```python
from build123d import *

# Parameters (mm, degrees)
CROQUIS1_R              = 2.5
SALIENTE_EXTRUIR1_DEPTH = 62
CORTAR_EXTRUIR1_DEPTH   = 17.5
CHAFL_N1_SIZE           = 0.2


with BuildPart() as part:
    # Croquis1 → Saliente-Extruir1 (new body)
    with BuildSketch(Plane(origin=(0, 0, 0), x_dir=(1, 0, 0), z_dir=(0, 1, 0))):
        Circle(CROQUIS1_R)
    extrude(amount=SALIENTE_EXTRUIR1_DEPTH)

    # Croquis2 → Cortar-Extruir1 (cut)
    with BuildSketch(Plane(origin=(0, 62, 0), x_dir=(1, 0, 0), z_dir=(0, 1, 0))):
        with BuildLine():
            Line((-1.920937271, 1.6), (1.920937271, 1.6))
            ThreePointArc((1.920937271, 1.6), (0, 2.5), (-1.920937271, 1.6))
        make_face()
    extrude(amount=-CORTAR_EXTRUIR1_DEPTH, mode=Mode.SUBTRACT)

    # Chaflán1
    chafl_n1_edges = [part.edges().sort_by_distance(p)[0] for p in [
        (-0.850781059, 62, 2.350781059),
        (-2.5, 0, 0),
    ]]
    chamfer(chafl_n1_edges, length=CHAFL_N1_SIZE)


solid = part.part
```
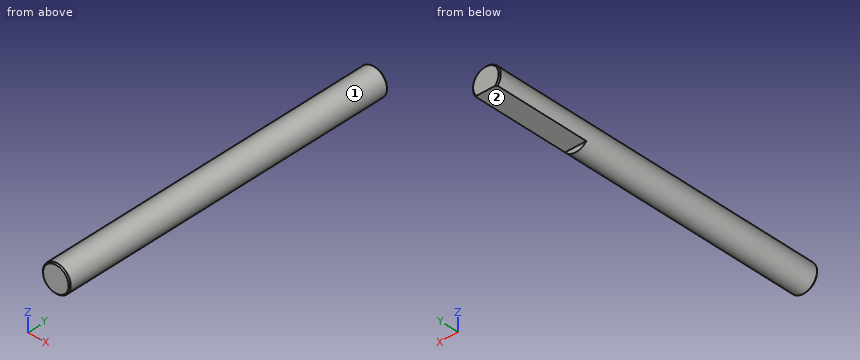
Verification items for the finished model (mm, model axes). Face numbers are marked on the shaded views. A direction names the side the tool comes from. Round coordinates to 2 decimals unless told otherwise and drop trailing zeros. Write each loop counter-clockwise with the first axis right and the second up, starting at its lowest first coordinate (ties: lowest second). Pieces come first, ordered by that corner, then holes.
1. Access from +Z, -Z, +X, -X, +Y, -Y to the whole of each face (thin tool, end or side, straight path). Record for the marked faces 1 and 2.
2. Section check B-B on y = 55.5. Enter the section's corners in (x, z).
3. Section check A-A on x = 0. Enter the section's corners in (y, z).
4. Gauge pin test, flat ends, axial feed: P1, Ø3, axis at x = 0.5, y = 52, coming from the -Z side; P2, Ø1, axis at y = 37, z = 1.5, coming from the -X side; P3, Ø0.5, axis at x = -0.5, z = -2, coming from the +Y side. Record the tip position at first contact, or that the pin passes through.
5. Section check C-C on y = 15.5. Enter the section's corners in (x, z).
6. Scan lines: L1, parallel to X at y = 23, z = -1.6; L2, parallel to X at y = 53.5, z = -0.2; L3, parallel to Z at x = 1.1, y = 59 (3 decimals). Record each from-to range of solid material in increasing order.
Answer:
1. face 1: +Y, -Y
1. face 2: -Z, +X, -X, +Y
2. outline: (-1.92, -1.6) - (1.92, -1.6) arc R2.5 ccw (long way) to start
3. outline: (0, -2.3) - (0.2, -2.5) - (44.5, -2.5) - (44.5, -1.6) - (62, -1.6) - (62, 2.3) - (61.8, 2.5) - (0.2, 2.5) - (0, 2.3) - close
4. P1: stops at z = -1.6
4. P2: stops at x = -2.29
4. P3: stops at y = 44.5
5. outline: circle Ø5 at (0, 0)
6. L1: x = -1.92 to 1.92
6. L2: x = -2.49 to 2.49
6. L3: z = -1.6 to 2.245
